from build123d import *

# Parameters (mm, degrees)
BOSS_EXTRUDE4_DEPTH = 20


with BuildPart() as part:
    # Sketch1 → Boss-Extrude4 (new body)
    with BuildSketch(Plane(origin=(0, 0, 0), x_dir=(1, 0, 0), z_dir=(0, 1, 0))):
        with BuildLine():
            Line((-55, -24.494897428), (-55, -19.364916731))
            ThreePointArc((-55, -19.364916731), (-70, 0), (-55, 19.364916731))
            Line((-55, 19.364916731), (-55, 24.494897428))
            ThreePointArc((-55, 24.494897428), (-75, 0), (-55, -24.494897428))
        make_face()
        with BuildLine():
            ThreePointArc((-55, 19.364916731), (-52.52008585, 19.840593925), (-50, 20))
            Line((-50, 20), (-35, 20))
            ThreePointArc((-35, 20), (-42.09430585, 23.717082451), (-50, 25))
            ThreePointArc((-50, 25), (-52.51272405, 24.873403825), (-55, 24.494897428))
            Line((-55, 24.494897428), (-55, 19.364916731))
        make_face()
        with BuildLine():
            ThreePointArc((-50, 25), (-42.09430585, 23.717082451), (-35, 20))
            Line((-35, 20), (35, 20))
            ThreePointArc((35, 20), (42.094305882, 23.717082462), (50.000000068, 25))
            Line((50.000000068, 25), (-50, 25))
        make_face()
        with BuildLine():
            ThreePointArc((50.000000068, 25), (42.094305882, 23.717082462), (35, 20))
            Line((35, 20), (50, 20))
            ThreePointArc((50, 20), (52.52008585, 19.840593925), (55, 19.364916731))
            Line((55, 19.364916731), (55, 24.494897428))
            ThreePointArc((55, 24.494897428), (52.512724084, 24.873403822), (50.000000068, 25))
        make_face()
        with BuildLine():
            ThreePointArc((70, 0), (65.811388301, -12.247448714), (55, -19.364916731))
            Line((55, -19.364916731), (55, -24.494897428))
            ThreePointArc((55, -24.494897428), (69.364916731, -15.811388301), (75, 0))
            ThreePointArc((75, 0), (69.364916731, 15.811388301), (55, 24.494897428))
            Line((55, 24.494897428), (55, 19.364916731))
            ThreePointArc((55, 19.364916731), (65.811388301, 12.247448714), (70, 0))
        make_face()
        with BuildLine():
            Line((50, -20), (35, -20))
            ThreePointArc((35, -20), (42.09430585, -23.717082451), (50, -25))
            ThreePointArc((50, -25), (52.51272405, -24.873403825), (55, -24.494897428))
            Line((55, -24.494897428), (55, -19.364916731))
            ThreePointArc((55, -19.364916731), (52.52008585, -19.840593925), (50, -20))
        make_face()
        with BuildLine():
            Line((-35, -20), (-50, -20))
            ThreePointArc((-50, -20), (-52.52008585, -19.840593925), (-55, -19.364916731))
            Line((-55, -19.364916731), (-55, -24.494897428))
            ThreePointArc((-55, -24.494897428), (-52.51272405, -24.873403825), (-50, -25))
            ThreePointArc((-50, -25), (-42.09430585, -23.717082451), (-35, -20))
        make_face()
        with BuildLine():
            Line((35, -20), (-35, -20))
            ThreePointArc((-35, -20), (-42.09430585, -23.717082451), (-50, -25))
            Line((-50, -25), (50, -25))
            ThreePointArc((50, -25), (42.09430585, -23.717082451), (35, -20))
        make_face()
    extrude(amount=BOSS_EXTRUDE4_DEPTH)


solid = part.part
Part model, mm, in its own coordinate system. A direction names the side the tool comes from. Coordinates: 2 decimals unless noted, no trailing zeros. Loops run counter-clockwise (first coordinate to the right, second up) from the corner with the lowest first, then second, coordinate; pieces in that order, holes last. Notation, with made-up numbers: (51, -22.5) - (71, -22.5) arc R25 cw to (71, -1.5) - close; hole circle Ø7 at (67, -37). An arc over 180 degrees is marked (long way). Write each question's results on one line, items separated by ' | '. Start each with the question number.
Q1. Slice it at C-C on y = 4. Give the cut face in (x, z).
Q2. Slice it at B-B on z = 7.5. Give the cut face in (x, y).
Q3. Two-plate mould, pull along Z, no slides. Class faces 1 (the flat face through (1, 10, 20)), 2 (the flat face through (-1, 10, 25)), 3 (the flat face through (-0.4, 0, 20.3)): +Z half, -Z half, draft (parallel to the pull), parting line (faces both ways), or undercut.
Q4. Probe line 1 along Z through (x, y) = (26, 18.25); line 2 along X through (y, z) = (18, -10); line 3 along Z through (x, y) = (64.5, 15.25). List the from-to ranges inside material, lowest first.
Q5. Drop a flat-ended pin along its axis: pin 1 Ø3 at (y, z) = (6.5, 4) entering from +X. Give the stop position or say it passes through.
Q6. Which spindle directions (+Z, -Z, +X, -X, +Y, -Y) get a long thin tool onto all of the face, cutting with end or side? Do faces 4 (the flat face through (-0.4, 20, 20.3)), 5 (the flat face through (-1, 10, -20)). Say none if no direction does.
Q7. Slice it at A-A on x = 45.5. Give the cut face in (y, z).
Answer:
1) outline: (-50, -25) - (50, -25) arc R25 ccw to (50, 25) - (-50, 25) arc R25 ccw to start; hole (-50, -20) - (50, -20) arc R20 ccw to (50, 20) - (-50, 20) arc R20 ccw to start
2) outline: (-73.85, 0) - (-68.54, 0) - (-68.54, 20) - (-73.85, 20) - close; (68.54, 0) - (73.85, 0) - (73.85, 20) - (68.54, 20) - close
3) face 1: undercut | face 2: +Z half | face 3: draft
4) line 1: z = -25 to -20, 20 to 25 | line 2: x = -72.91 to -67.32, 67.32 to 72.91 | line 3: z = -20.37 to -13.77, 13.77 to 20.37
5) pin 1: stops at x = 74.87
6) face 4: +Z, -Z, +X, -X, +Y | face 5: +Y, -Y
7) outline: (0, -25) - (20, -25) - (20, -20) - (0, -20) - close; (0, 20) - (20, 20) - (20, 25) - (0, 25) - close
